from build123d import *

# Parameters (mm, degrees)
BOSS_EXTRUDE1_DEPTH = 6
BOSS_EXTRUDE2_DEPTH = 5
CHAMFER1_SIZE       = 5
SKETCH3_W           = 10
SKETCH3_H           = 3
CUT_EXTRUDE1_DEPTH  = 6


with BuildPart() as part:
    # Sketch1 → Boss-Extrude1 (new body)
    with BuildSketch(Plane.XY):
        with BuildLine():
            Line((-0.533466094, 0), (-3.5, 0))
            Line((-3.5, 0), (-3.5, -5))
            Line((-3.5, -5), (0, -5))
            add(Edge.make_bspline(
                [(0, -5), (42.604817908, 29.035673618), (94.903787643, 20)],
                knots=[0, 0, 0, 1, 1, 1], degree=2))
            Line((94.903787643, 20), (101.903787643, 20))
            Line((101.903787643, 20), (125.469317842, 44.504980705))
            Line((125.469317842, 44.504980705), (142.489368048, 44.504980705))
            Line((142.489368048, 44.504980705), (142.489368048, -10))
            Line((142.489368048, -10), (147.489368048, -10))
            Line((147.489368048, -10), (147.489368048, -7))
            Line((147.489368048, -7), (149.489368048, -7))
            Line((149.489368048, -7), (149.489368048, 51.504980705))
            Line((149.489368048, 51.504980705), (122.489368048, 51.504980705))
            Line((122.489368048, 51.504980705), (98.295822857, 26.346948908))
            add(Edge.make_bspline(
                [(-0.533451554, 1.707670566), (28.799887609, 25.188101284), (61.717873648, 33.515524554), (98.026818716, 26.400472635), (98.295822857, 26.346948908)],
                knots=[0, 0, 0, 0, 1, 1.00745886, 1.00745886, 1.00745886, 1.00745886], degree=3))
            Line((-0.533451554, 1.707670566), (-0.533466094, 0))
        make_face()
    extrude(amount=BOSS_EXTRUDE1_DEPTH)

    # Sketch2 → Boss-Extrude2 (add)
    with BuildSketch(Plane.XY.offset(6)):
        Polygon((149.489368048, -7), (157.267488672, -7), (149.489368048, 13.763788313), align=None)
    extrude(amount=-BOSS_EXTRUDE2_DEPTH)

    # Chamfer1
    chamfer1_edges = [part.edges().sort_by_distance(p)[0] for p in [
        (142.489368048, 44.504980705, 3),
    ]]
    chamfer(chamfer1_edges, length=CHAMFER1_SIZE)

    # Sketch3 → Cut-Extrude1 (cut)
    with BuildSketch(Plane.XY.offset(6)):
        with Locations((134.74873736, 48.004980705)):
            Rectangle(SKETCH3_W, SKETCH3_H)
    extrude(amount=-CUT_EXTRUDE1_DEPTH, mode=Mode.SUBTRACT)


solid = part.part
Part model, mm, in its own coordinate system. A direction names the side the tool comes from. Coordinates: 2 decimals unless noted, no trailing zeros. Loops run counter-clockwise (first coordinate to the right, second up) from the corner with the lowest first, then second, coordinate; pieces in that order, holes last. Notation, with made-up numbers: (-16, -14) - (11, -14) arc R13 ccw to (11, -9) - close; hole circle Ø5 at (-17.75, -12.5). An arc over 180 degrees is marked (long way). Write each question's results on one line, items separated by ' | '. Start each with the question number.
Q1. Drop flat-ended pins along their axis: pin 1 Ø3.5 at (x, z) = (-2.5, 2) entering from +Y; pin 2 Ø3 at (y, z) = (18, 5) entering from -X; pin 3 Ø1.8 at (x, z) = (-1, 3.5) entering from -Y. Give the stop position or say it passes through.
Q2. Slice it at A-A on y = 38. Give the cut face in (x, z), and give its area (3 significant figures).
Q3. Probe line 1 along Y through (x, z) = (134, 2); line 2 along X through (y, z) = (-2.5, 3); line 3 along X through (y, z) = (29.5, 3). List the from-to ranges inside material, lowest first.
Q4. Two-plate mould, pull along X, no slides. Class faces 1 (the flat face through (142.489, 15, 3)), 2 (the flat face through (140.024, 41.97, 2.958)), 3 (the flat face through (149.489, 28, 3)), 4 (the flat face through (152, -7, 3)): +X half, -X half, draft (parallel to the pull), parting line (faces both ways), or undercut.
Q5. Which spindle directions (+Z, -Z, +X, -X, +Y, -Y) get a long thin tool onto all of the face, cutting with end or side? Do faces 5 (the flat face through (98, 20, 3)), 6 (the flat face through (147.489, -9, 3)), 7 (the flat face through (129.749, 48, 3)), 8 (the flat face through (-2, 0, 3)), 9 (the flat face through (-2, -5, 3)). Say none if no direction does.
Answer:
1) pin 1: stops at y = 0 | pin 2: stops at x = 22.16 | pin 3: stops at y = -5
2) outline: (109.5, 0) - (119.21, 0) - (119.21, 6) - (109.5, 6) - close; (142.49, 0) - (149.49, 0) - (149.49, 6) - (142.49, 6) - close | area: 100 mm2
3) line 1: y = 44.5 to 46.5, 49.5 to 51.5 | line 2: x = -3.5 to 3.22, 142.49 to 155.58 | line 3: x = 101.33 to 111.04, 142.49 to 149.49
4) face 1: undercut | face 2: undercut | face 3: +X half | face 4: draft
5) face 5: +Z, -Z, -Y | face 6: +Z, -Z, +X, -Y | face 7: +Z, -Z | face 8: +Z, -Z, -X, +Y | face 9: +Z, -Z, -X, -Y
